Verification items for the finished model (mm, model axes). A direction names the side the tool comes from. Round coordinates to 2 decimals unless told otherwise and drop trailing zeros. Loops run counter-clockwise (first coordinate to the right, second up) from the corner with the lowest first, then second, coordinate; pieces in that order, holes last. Notation, with made-up numbers: (-15.5, 25.5) -> (43.5, 25.5) arc R21 cw to (43.5, 44.5) -> close; hole circle Ø9 at (50.5, 43). An arc over 180 degrees is marked (long way). Write item = value, one per line.
```python
from build123d import *

# Parameters (mm, degrees)
SKETCH1_W           = 39
SKETCH1_H           = 62
BOSS_EXTRUDE1_DEPTH = 2
BOSS_EXTRUDE2_DEPTH = 11


with BuildPart() as part:
    # Sketch1 → Boss-Extrude1 (new body)
    with BuildSketch(Plane(origin=(0, 0, 0), x_dir=(1, 0, 0), z_dir=(0, 1, 0))):
        Polygon((0.5, 29), (-0.5, 29), (-0.5, -33), (-39.5, -33), (-39.5, 29), (-31.5, 29), (-31.5, 30), (-39.5, 30), (-39.5, 33), (25.5, 33), (25.5, 34), (-40.5, 34), (-40.5, -34), (40.5, -34), (40.5, 30), (31.5, 30), (31.5, 29), (39.5, 29), (39.5, -33), (0.5, -33), align=None)
        Polygon((-31.5, 29), (-8.5, 29), (-8.5, 30), (8.5, 30), (8.5, 29), (31.5, 29), (31.5, 30), (40.5, 30), (40.5, 34), (25.5, 34), (25.5, 33), (-39.5, 33), (-39.5, 30), (-31.5, 30), align=None)
        with Locations((-20, -2)):
            Rectangle(SKETCH1_W, SKETCH1_H)
        with Locations((20, -2)):
            Rectangle(SKETCH1_W, SKETCH1_H)
        Polygon((-8.5, 29), (-0.5, 29), (0.5, 29), (8.5, 29), (8.5, 30), (-8.5, 30), align=None)
    extrude(amount=-BOSS_EXTRUDE1_DEPTH)

    # Sketch1_3 → Boss-Extrude2 (add)
    with BuildSketch(Plane(origin=(0, 0, 0), x_dir=(1, 0, 0), z_dir=(0, 1, 0))):
        Polygon((0.5, 29), (-0.5, 29), (-0.5, -33), (-39.5, -33), (-39.5, 29), (-31.5, 29), (-31.5, 30), (-39.5, 30), (-39.5, 33), (25.5, 33), (25.5, 34), (-40.5, 34), (-40.5, -34), (40.5, -34), (40.5, 30), (31.5, 30), (31.5, 29), (39.5, 29), (39.5, -33), (0.5, -33), align=None)
    extrude(amount=BOSS_EXTRUDE2_DEPTH)


solid = part.part
```
(1) Sectioned sample at B-B, the plane y = 1.5. Record the cut outline in (x, z), and give its area (3 significant figures).
Filled sheet:
outline = (-40.5, -34) -> (25.5, -34) -> (25.5, -33) -> (-39.5, -33) -> (-39.5, -30) -> (-31.5, -30) -> (-31.5, -29) -> (-39.5, -29) -> (-39.5, 33) -> (-0.5, 33) -> (-0.5, -29) -> (0.5, -29) -> (0.5, 33) -> (39.5, 33) -> (39.5, -29) -> (31.5, -29) -> (31.5, -30) -> (40.5, -30) -> (40.5, 34) -> (-40.5, 34) -> close
area = 354 mm2
(2) Material ranges on probe 1 along X at (y, z) = (6.5, -7.5); probe 2 along Z at (x, y) = (32.5, 5.25); probe 3 along Z at (x, y) = (-19.5, 1.5), recorded low to high. Write a range as from..to.
Filled sheet:
probe_1 = -40.5..-39.5, -0.5..0.5, 39.5..40.5
probe_2 = -30..-29, 33..34
probe_3 = -34..-33, 33..34
(3) Set-up check for faces 1 (the face through (0, 11, 2)), 2 (the face through (36, 5, -30)), 3 (the face through (-20, 5, 33)), 4 (the face through (-35, 5, -30)): record each of +Z, -Z, +X, -X, +Y, -Y from which the full face is reachable in a straight line by a thin tool's end or side.
Filled sheet:
face_1 = +Z, -Z, +X, -X, +Y
face_2 = -Z, +X, +Y
face_3 = +Y
face_4 = +X, +Y
(4) Sectioned sample at D-D, the plane x = 7.5. Record the cut outline in (y, z), and give its area (3 significant figures).
Filled sheet:
outline = (-2, -34) -> (11, -34) -> (11, -33) -> (0, -33) -> (0, 33) -> (11, 33) -> (11, 34) -> (-2, 34) -> close
area = 158 mm2
(5) Sectioned sample at C-C, the plane z = 9.5. Record the cut outline in (x, y), and give its area (3 significant figures).
Filled sheet:
outline = (-40.5, -2) -> (40.5, -2) -> (40.5, 11) -> (39.5, 11) -> (39.5, 0) -> (0.5, 0) -> (0.5, 11) -> (-0.5, 11) -> (-0.5, 0) -> (-39.5, 0) -> (-39.5, 11) -> (-40.5, 11) -> close
area = 195 mm2
(6) Draft check along Z on faces 5 (the face through (-36, 5, -29)), 6 (the face through (-1, 4, 34)), 7 (the face through (-40.5, 4, 0)). Enter one of: released by +Z, released by -Z, zero draft, split by the parting line, or undercut.
Filled sheet:
face_5 = undercut
face_6 = released by +Z
face_7 = zero draft
(7) Go/stop test with flat-tipped pins: pin 1 Ø4.5 at (x, y) = (34, 6.5) entering from -Z; pin 2 Ø3 at (x, z) = (20.5, -26) entering from +Y. Record where each tip stops, or that it passes through.
Filled sheet:
pin_1 = -30
pin_2 = 0
(8) Sectioned sample at A-A, the plane x = 30.5. Record the cut outline in (y, z).
Filled sheet:
outline = (-2, -34) -> (0, -34) -> (0, 33) -> (11, 33) -> (11, 34) -> (-2, 34) -> close
